Work out the finished part from the listing and answer in its coordinate system (mm). A direction names the side the tool comes from. Give positions to 0.01 mm unless a question says otherwise; leave off trailing zeros. Loops run counter-clockwise (first coordinate to the right, second up) from the corner with the lowest first, then second, coordinate; pieces in that order, holes last. Notation, with made-up numbers: (12, -28.75) - (25, -28.75) arc R26 ccw to (25, -2.75) - close; hole circle Ø11 at (61, 7.25). An arc over 180 degrees is marked (long way). One line per question, with ' | ' between items. Start each with the question number.
1. Each of these flat-tipped pins is pushed along its axis until it touches: pin 1 (1.7 mm diameter, centred on x = -0.5, z = 65.5, fed in from +Y); pin 2 (2 mm diameter, centred on x = 3, y = 4.5, fed in from -Z); pin 3 (6 mm diameter, centred on x = 12.5, z = 16, fed in from +Y); pin 4 (3 mm diameter, centred on x = 13, z = 7.5, fed in from -Y). Where does it stop, or does it pass through?
2. Find the intervals of material crossed by line 1 (Y direction, x = 0, z = 63); line 2 (Z direction, x = 3, y = -1); line 3 (Y direction, x = 0, z = 25.5), in increasing order.
3. Section A-A (x = 0) is taken. Determine the outline of the cut face in (y, z), plus the area to 3 significant figures.
4. Section D-D (x = -8.5) is taken. Determine the outline of the cut face in (y, z).
5. Which of the six approach directions +Z, -Z, +X, -X, +Y, -Y give full straight-line access (tool end or side, diameter ignored) to faces 1 (the face through (0, 2.5, 64)), 2 (the face through (0, 0, 71))?
6. Section B-B (y = 9) is taken. Determine the outline of the cut face in (x, z).
7. Section C-C (z = 52) is taken. Determine the outline of the cut face in (x, y).
from build123d import *

# Parameters (mm, degrees)
SKETCH1_R           = 18.5
BOSS_EXTRUDE1_DEPTH = 57
BOSS_EXTRUDE2_DEPTH = 14


with BuildPart() as part:
    # Sketch1 → Boss-Extrude1 (new body)
    with BuildSketch(Plane.XY):
        Circle(SKETCH1_R)
    extrude(amount=BOSS_EXTRUDE1_DEPTH)

    # Sketch2 → Boss-Extrude2 (add)
    with BuildSketch(Plane.XY.offset(57)):
        with BuildLine():
            Line((1.658312395, 2.5), (-1.658312395, 2.5))
            ThreePointArc((-1.658312395, 2.5), (-1.418637165, -2.643382037), (3, 0))
            ThreePointArc((3, 0), (2.643382037, 1.418637165), (1.658312395, 2.5))
        make_face()
    extrude(amount=BOSS_EXTRUDE2_DEPTH)


solid = part.part
Conclusion:
1) pin 1: y = 2.5 | pin 2: z = 0 | pin 3: y = 15.87 | pin 4: y = -14.49
2) line 1: -3 to 2.5 | line 2: 0 to 57 | line 3: -18.5 to 18.5
3) outline: (-18.5, 0) - (18.5, 0) - (18.5, 57) - (2.5, 57) - (2.5, 71) - (-3, 71) - (-3, 57) - (-18.5, 57) - close | area: 2,190 mm²
4) outline: (-16.43, 0) - (16.43, 0) - (16.43, 57) - (-16.43, 57) - close
5) face 1: +Z, +X, -X, +Y | face 2: +Z, +X, -X, +Y, -Y
6) outline: (-16.16, 0) - (16.16, 0) - (16.16, 57) - (-16.16, 57) - close
7) outline: circle Ø37 at (0, 0)
